Geometry: final body of the model. Coordinates: model frame, mm. Round coordinates to 2 decimals unless told otherwise and drop trailing zeros. Loops run counter-clockwise (first coordinate to the right, second up) from the corner with the lowest first, then second, coordinate; pieces in that order, holes last. Notation, with made-up numbers: (48, 63) -> (52, 63) arc R19 ccw to (52, 100) -> close; hole circle Ø7 at (-35, 65.5). An arc over 180 degrees is marked (long way). Answer in a Markdown table with one row per item.
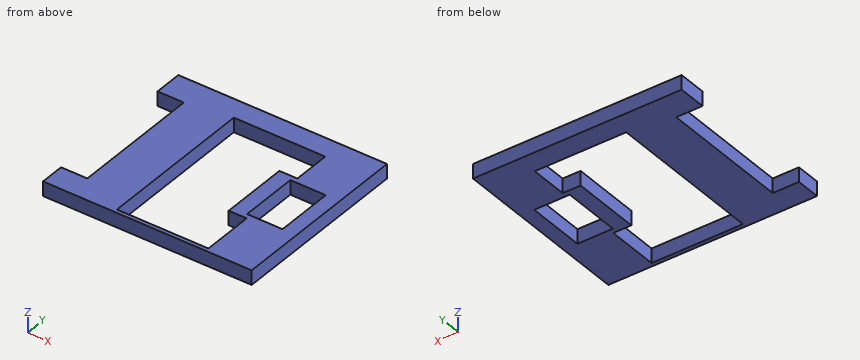
```python
from build123d import *

# Parameters (mm, degrees)
F0_W     = 20.54
F0_H     = 18.09
F0_W_2   = 2.57
F0_H_2   = 12.9
F0_W_3   = 3.49
F0_H_3   = 5.78
F1_DEPTH = 1.42
F2_W     = 0.015
F2_H     = 12.9
F3_DEPTH = 1.421


with BuildPart() as f1:
    # F0 (on Top) → F1 (new body)
    with BuildSketch(Plane.XY):
        with Locations((10.27, 9.045)):
            Rectangle(F0_W, F0_H)
        with Locations((1.3, 8.86)):
            Rectangle(F0_W_2, F0_H_2, mode=Mode.SUBTRACT)
        Polygon((7, 0.38), (7, 16), (16, 16), (16, 12.27), (14.23, 12.27), (14.23, 5.5), (16, 5.5), (16, 0.38), align=None, mode=Mode.SUBTRACT)
        with Locations((17.42, 8.88)):
            Rectangle(F0_W_3, F0_H_3, mode=Mode.SUBTRACT)
    extrude(amount=F1_DEPTH)

    # F2 (on face) → F3 (cut, through all)
    with BuildSketch(Plane.XY.offset(1.42)):
        with Locations((0.0075, 8.86)):
            Rectangle(F2_W, F2_H)
    extrude(amount=-F3_DEPTH, mode=Mode.SUBTRACT)


solid = f1.part
```
Item 1: Cut plane B-B (z = 0.5). Output: boundary loops of the cut face in (x, y) (3 decimals), then the cut area to 3 significant figures.
Answer:
| item | result |
|---|---|
| outline | (0, 0) -> (20.54, 0) -> (20.54, 18.09) -> (0, 18.09) -> (0, 15.31) -> (2.585, 15.31) -> (2.585, 2.41) -> (0, 2.41) -> close; hole (7, 0.38) -> (16, 0.38) -> (16, 5.5) -> (14.23, 5.5) -> (14.23, 12.27) -> (16, 12.27) -> (16, 16) -> (7, 16) -> close; hole (15.675, 5.99) -> (19.165, 5.99) -> (19.165, 11.77) -> (15.675, 11.77) -> close |
| area | 189 mm² |
Item 2: Cut plane D-D (y = 13.75). Output: boundary loops of the cut face in (x, z) (3 decimals), then the cut area to 3 significant figures.
Answer:
| item | result |
|---|---|
| outline | (2.585, 0) -> (7, 0) -> (7, 1.42) -> (2.585, 1.42) -> close; (16, 0) -> (20.54, 0) -> (20.54, 1.42) -> (16, 1.42) -> close |
| area | 12.7 mm² |
Item 3: Pin query (flat end, axial travel): pin 1 Ø0.7 at (y, z) = (8.5, 1) entering from -X (3 decimals). Return the tip coordinate at first contact, or that it passes through.
Answer:
| item | result |
|---|---|
| pin 1 | stops at x = 2.585 |
Item 4: Line query: probe 1 along X at (y, z) = (7, 0.8) (3 decimals); probe 2 along Y at (x, z) = (7.25, 1.05); probe 3 along X at (y, z) = (12, 1.25) (3 decimals). Output: solid intervals per line, ascending. Write a range as [from, to].
Answer:
| item | result |
|---|---|
| probe 1 | x = [2.585, 7], [14.23, 15.675], [19.165, 20.54] |
| probe 2 | y = [0, 0.38], [16, 18.09] |
| probe 3 | x = [2.585, 7], [14.23, 20.54] |
Item 5: Cut plane A-A (x = 1.5). Output: boundary loops of the cut face in (y, z).
Answer:
| item | result |
|---|---|
| outline | (0, 0) -> (2.41, 0) -> (2.41, 1.42) -> (0, 1.42) -> close; (15.31, 0) -> (18.09, 0) -> (18.09, 1.42) -> (15.31, 1.42) -> close |
Item 6: Cut plane C-C (y = 6.25). Output: boundary loops of the cut face in (x, z) (3 decimals).
Answer:
| item | result |
|---|---|
| outline | (2.585, 0) -> (7, 0) -> (7, 1.42) -> (2.585, 1.42) -> close; (14.23, 0) -> (15.675, 0) -> (15.675, 1.42) -> (14.23, 1.42) -> close; (19.165, 0) -> (20.54, 0) -> (20.54, 1.42) -> (19.165, 1.42) -> close |
